Part print with two shaded views. Sizes in mm from the minimum x, y, z corner. Round coordinates to 2 decimals unless told otherwise and drop trailing zeros. Order: outer loops, then holes, each group sorted by start corner. A loop starts at its lowest first (then second) coordinate and runs counter-clockwise, first axis right, second up. Notation, with made-up numbers: (79, 58) -> (126, 58) arc R19 cw to (126, 86) -> close; hole circle Ø2 at (-17, 57). An arc over 180 degrees is marked (long way). Put each result on its own line as item: value. Start each with the question number.
Q1. Cut at D-D, the plane x = 5. List the corners of the cut face in (y, z).
Q2. Probe L1, parallel to Y at x = 35, z = 9; L2, parallel to Y at x = 35, z = 28. List the from-to ranges inside material, lowest first.
Q3. Cut at A-A, the plane y = 35. List the corners of the cut face in (x, z).
Q4. Cut at C-C, the plane z = 16. List the corners of the cut face in (x, y).
Q5. Flat gauge pins, fed straight in: P1, Ø5, axis at y = 40, z = 10.5, coming from the -X side; P2, Ø5, axis at y = 58, z = 27, coming from the +X side; P3, Ø6, axis at x = 29, y = 12, coming from the -Z side; P4, Ø4, axis at x = 29, z = 17.5, coming from the -Y side. Where does each tip first touch, or does it go through?
Q6. Pull direction Y, two halves, no side cores. Call the marked faces 1, 2 and 3: released by +Y, released by -Y, zero draft, split by the parting line, or undercut.
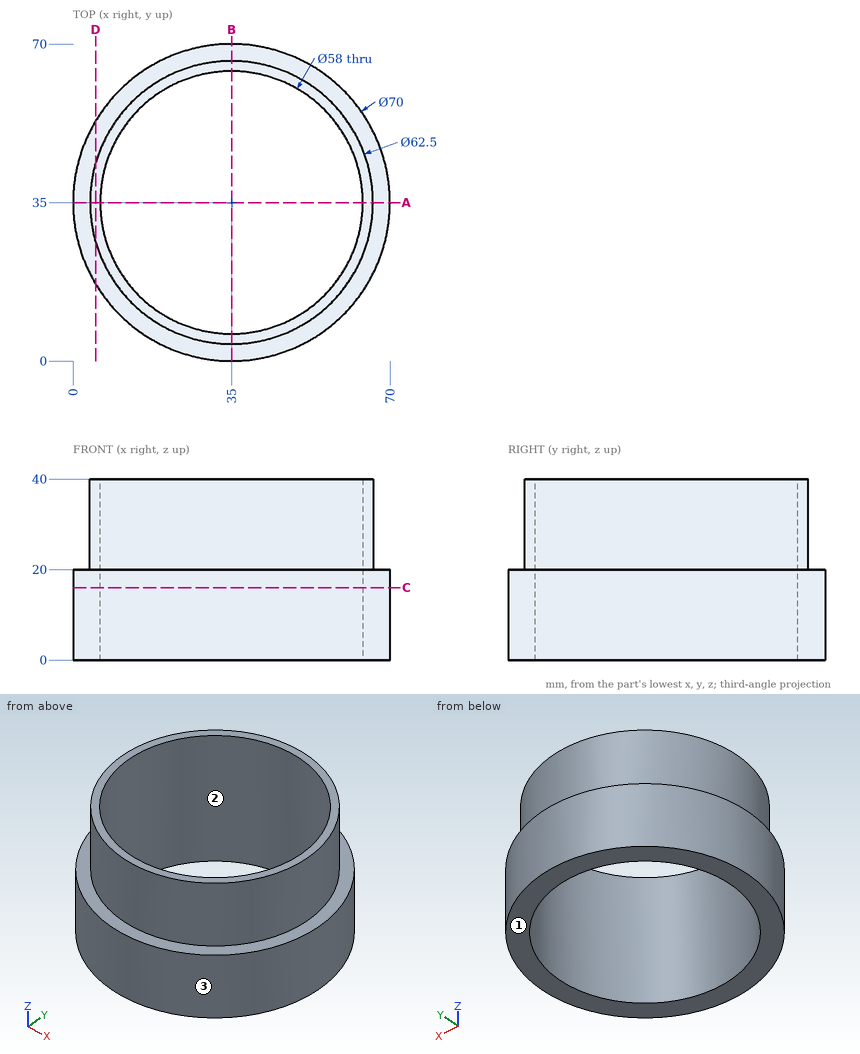
Ans:
1. outline: (16.97, 0) -> (53.03, 0) -> (53.03, 20) -> (43.75, 20) -> (43.75, 40) -> (26.25, 40) -> (26.25, 20) -> (16.97, 20) -> close
2. L1: y = 0 to 6, 64 to 70
2. L2: y = 3.75 to 6, 64 to 66.25
3. outline: (0, 0) -> (6, 0) -> (6, 40) -> (3.75, 40) -> (3.75, 20) -> (0, 20) -> close; (64, 0) -> (70, 0) -> (70, 20) -> (66.25, 20) -> (66.25, 40) -> (64, 40) -> close
4. outline: circle Ø70 at (35, 35); hole circle Ø58 at (35, 35)
5. P1: stops at x = 0.09
5. P2: stops at x = 58.59
5. P3: passes through
5. P4: stops at y = 0.23
6. face 1: zero draft
6. face 2: undercut
6. face 3: split by the parting line
